```python
from build123d import *

# Parameters (mm, degrees)
F1_DEPTH = 430
F2_W     = 128
F2_H     = 8.4
F3_DEPTH = 7
F5_DEPTH = 430


with BuildPart() as f1:
    # F0 (on Front) → F1 (new body)
    with BuildSketch(Plane.XZ):
        Polygon((-47.436745, 38.990075), (-57.436745, 38.990075), (-57.436745, 36.490075), (-54.436745, 36.490075), (-54.436745, 33.090075), (-56.436745, 33.090075), (-56.436745, 30.590075), (-47.436745, 30.590075), align=None)
    extrude(amount=F1_DEPTH)

    # F2 (on Front) → F3 (join)
    with BuildSketch(Plane.XZ):
        with Locations((-111.436745, 34.790075)):
            Rectangle(F2_W, F2_H)
    extrude(amount=-F3_DEPTH)

    # F4 (on Front) → F5 (join)
    with BuildSketch(Plane.XZ):
        Polygon((-165.436745, 36.57085), (-165.436745, 39.07085), (-175.436745, 39.07085), (-175.436745, 30.67085), (-166.436745, 30.67085), (-166.436745, 33.17085), (-168.436745, 33.17085), (-168.436745, 36.57085), align=None)
    extrude(amount=F5_DEPTH)


solid = f1.part
```
Work out the finished part from the listing and answer in its coordinate system (mm). Give positions to 0.01 mm unless a question says otherwise; leave off trailing zeros. Loops run counter-clockwise (first coordinate to the right, second up) from the corner with the lowest first, then second, coordinate; pieces in that order, holes last. Notation, with made-up numbers: (59, -36.75) -> (109, -36.75) arc R18 cw to (109, -6.75) -> close; hole circle Ø5 at (39, -32). An arc over 180 degrees is marked (long way). Write item = value, one per line. Start each with the question number.
(1) Find section A-A on y = -42. Give the vertices of the cut face in (x, z), and give its area (3 significant figures).
(2) Given pin 1 Ø2.5 at (x, y) = (-167, -214.5) entering from -Z; pin 2 Ø2 at (x, z) = (-155, 33.5) entering from -Y; pin 3 Ø0.6 at (x, y) = (-55, -195) entering from +Z, each flat-ended and moving along its own axis, determine where each tip first touches the part or whether it passes through.
(3) Find the intervals of material crossed by probe 1 along X at (y, z) = (-208.5, 34.75); probe 2 along X at (y, z) = (-86.5, 32); probe 3 along Y at (x, z) = (-135, 37), in increasing order. Write a range as from..to.
(4) Find section B-B on x = -151.5. Give the vertices of the cut face in (y, z), and give its area (3 significant figures).
(5) The mould has two halves that part along X. Classify faces 1 (the flat face through (-102, 0, 35)), 2 (the flat face through (-172, -430, 35)), 3 (the flat face through (-175.437, -208, 35)): +X half, -X half, draft (parallel to the pull), parting line (faces both ways), or undercut.
From the geometry:
q1.outline = (-175.44, 30.67) -> (-166.44, 30.67) -> (-166.44, 33.17) -> (-168.44, 33.17) -> (-168.44, 36.57) -> (-165.44, 36.57) -> (-165.44, 39.07) -> (-175.44, 39.07) -> close; (-57.44, 36.49) -> (-54.44, 36.49) -> (-54.44, 33.09) -> (-56.44, 33.09) -> (-56.44, 30.59) -> (-47.44, 30.59) -> (-47.44, 38.99) -> (-57.44, 38.99) -> close
q1.area = 143 mm^2
q2.pin_1 = 30.67
q2.pin_2 = 0
q2.pin_3 = 38.99
q3.probe_1 = -175.44..-168.44, -54.44..-47.44
q3.probe_2 = -175.44..-166.44, -56.44..-47.44
q3.probe_3 = 0..7
q4.outline = (0, 30.59) -> (7, 30.59) -> (7, 38.99) -> (0, 38.99) -> close
q4.area = 58.8 mm^2
q5.face_1 = undercut
q5.face_2 = draft
q5.face_3 = -X half
